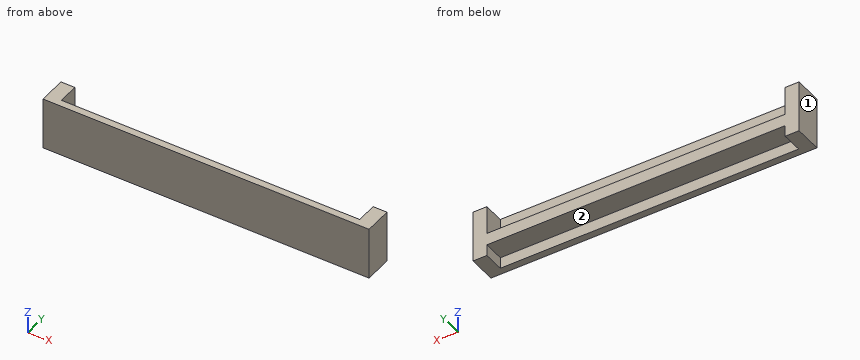
from build123d import *

# Parameters (mm, degrees)
BOSS_EXTRUDE1_DEPTH = 6
SKETCH2_W           = 94
SKETCH2_H           = 15
BOSS_EXTRUDE2_DEPTH = 2


with BuildPart() as part:
    # Sketch1 → Boss-Extrude1 (new body)
    with BuildSketch(Plane(origin=(0, 0, 0), x_dir=(1, 0, 0), z_dir=(0, 1, 0))):
        Polygon((57.138726824, 8.469222481), (61.138726824, 8.469222481), (61.138726824, 5.219222481), (147.138726824, 5.219222481), (147.138726824, 8.469222481), (151.138726824, 8.469222481), (151.138726824, -6.530777519), (147.138726824, -6.530777519), (147.138726824, 1.719222481), (61.138726824, 1.719222481), (61.138726824, -6.530777519), (57.138726824, -6.530777519), align=None)
    extrude(amount=BOSS_EXTRUDE1_DEPTH)

    # Sketch2 → Boss-Extrude2 (add)
    with BuildSketch(Plane.XZ):
        with Locations((104.138726824, -0.969222481)):
            Rectangle(SKETCH2_W, SKETCH2_H)
    extrude(amount=BOSS_EXTRUDE2_DEPTH)


solid = part.part
For this review, take the finished solid that the model builds, in its own axes (mm). Face numbers are marked on the shaded views. A direction names the side the tool comes from. Give positions to 0.01 mm unless a question says otherwise; leave off trailing zeros. Loops run counter-clockwise (first coordinate to the right, second up) from the corner with the lowest first, then second, coordinate; pieces in that order, holes last. Notation, with made-up numbers: (-12, 55.5) -> (47, 55.5) arc R18 cw to (47, 72.5) -> close; hole circle Ø8 at (-40, 68.25). An arc over 180 degrees is marked (long way). One line per question, with ' | ' between items.
1) To check wall thickness, follow probe 1 along X at (y, z) = (2, 5.5); probe 2 along Y at (x, z) = (123.5, -5.25); probe 3 along Z at (x, y) = (101, 5.75). State the ranges of each line that lie inside material, in increasing order.
Resolved:
probe 1: x = 57.14 to 61.14, 147.14 to 151.14 | probe 2: y = -2 to 0 | probe 3: z = -5.22 to -1.72
2) For the marked faces 1 and 2, list the 3-axis set-ups (+Z, -Z, +X, -X, +Y, -Y) from which the entire face can be reached by the end or side of a thin tool; tool diameter is ignored.
Resolved:
face 1: +Z, -Z, -X, +Y, -Y | face 2: -Z, +Y
3) Insertion check: pin 1 Ø1 at (x, z) = (92.5, -6) entering from +Y; pin 2 Ø1 at (x, y) = (82, 2) entering from -Z. Each pin has a flat end and moves straight along its axis. Give the tip position at first contact, or say it passes through.
Resolved:
pin 1: stops at y = 0 | pin 2: stops at z = -5.22
4) We need section C-C (x = 105.5). Write out the cut boundary in (y, z).
Resolved:
outline: (-2, -8.47) -> (0, -8.47) -> (0, -5.22) -> (6, -5.22) -> (6, -1.72) -> (0, -1.72) -> (0, 6.53) -> (-2, 6.53) -> close
5) We need section A-A (y = 2.25). Write out the cut boundary in (x, z).
Resolved:
outline: (57.14, -8.47) -> (61.14, -8.47) -> (61.14, -5.22) -> (147.14, -5.22) -> (147.14, -8.47) -> (151.14, -8.47) -> (151.14, 6.53) -> (147.14, 6.53) -> (147.14, -1.72) -> (61.14, -1.72) -> (61.14, 6.53) -> (57.14, 6.53) -> close
6) We need section B-B (z = 1.5). Write out the cut boundary in (x, y).
Resolved:
outline: (57.14, -2) -> (151.14, -2) -> (151.14, 6) -> (147.14, 6) -> (147.14, 0) -> (61.14, 0) -> (61.14, 6) -> (57.14, 6) -> close
